Geometry check sheet. Reference: the model listing, model coordinates, mm. Face numbers are marked on the shaded views. A direction names the side the tool comes from. Round coordinates to 2 decimals unless told otherwise and drop trailing zeros. Write each loop counter-clockwise with the first axis right and the second up, starting at its lowest first coordinate (ties: lowest second). Pieces come first, ordered by that corner, then holes. Notation, with made-up numbers: M 57.5,-3 L 72.5,-3 A30 ccw 72.5,19 Z; hole C 53.25,-20 d5. An arc over 180 degrees is marked long. Put each result on its own line as item: value. Start each with the question number.
(1) Gauge pin test, flat ends, axial feed: pin 1 (11.5 mm diameter, centred on x = 48.26, z = -48.26, fed in from +Y); pin 2 (20.5 mm diameter, centred on x = 48.26, z = 48.26, fed in from +Y); pin 3 (19 mm diameter, centred on y = 23, z = -13, fed in from +X). Record the tip position at first contact, or that the pin passes through.
(2) Tool access check on the marked faces 1, 2 and 3. Record the directions out of +Z, -Z, +X, -X, +Y, -Y that give a thin tool (end or side, any length) a straight path to the whole face; none if there is none.
(3) Material ranges on probe 1 along Z at (x, y) = (48.26, -9.75); probe 2 along X at (y, z) = (45.5, 20), recorded low to high.
(4) Section check A-A on x = -48.26. Record the cut outline in (y, z).
(5) Section check C-C on z = -24. Record the cut outline in (x, y).
(6) Section check B-B on y = -9.5. Record the cut outline in (x, z), then the cut area to 3 significant figures.
(7) Mould release check, pull along Z, two halves, no side actions. Record for the marked faces 4, 5 and 6: pulls with the +Z half, pulls with the -Z half, needs draft (parallel to the pull), parting line crosses it, or undercut.
(8) Section check D-D on x = -21. Record the cut outline in (y, z).
from build123d import *

# Parameters (mm, degrees)
SKETCH1_W          = 127
SKETCH1_H          = 127
EXTRUDE1_DEPTH     = 19.05
EXTRUDE2_DEPTH     = 38.1
SKETCH3_R          = 12.7
CUT_EXTRUDE1_DEPTH = 38.1
SKETCH4_W          = 38.1
SKETCH4_H          = 63.5
CUT_EXTRUDE2_DEPTH = 38.1
CUT_EXTRUDE3_REACH = 21.05
SKETCH5_R          = 6.35
CUT_EXTRUDE4_REACH = 21.05
SKETCH6_R          = 6.35
CUT_EXTRUDE5_REACH = 21.05
SKETCH8_R          = 6.35


with BuildPart() as part:
    # Sketch1 → Extrude1 (new body)
    with BuildSketch(Plane(origin=(0, 0, 0), x_dir=(1, 0, 0), z_dir=(0, 1, 0))):
        Rectangle(SKETCH1_W, SKETCH1_H)
    extrude(amount=-EXTRUDE1_DEPTH)

    # Sketch2 → Extrude2 (add, symmetric)
    with BuildSketch(Plane(origin=(0, 0, 0), x_dir=(0, 0, -1), z_dir=(1, 0, 0))):
        Polygon((38.1, 0), (26.903236725, 63.5), (-26.903236725, 63.5), (-38.1, 0), align=None)
    extrude(amount=EXTRUDE2_DEPTH, both=True)

    # Sketch3 → Cut-Extrude1 (cut, symmetric)
    with BuildSketch(Plane(origin=(0, 0, 0), x_dir=(0, 0, -1), z_dir=(1, 0, 0))):
        with Locations((0, 31.75)):
            Circle(SKETCH3_R)
    extrude(amount=CUT_EXTRUDE1_DEPTH, both=True, mode=Mode.SUBTRACT)

    # Sketch4 → Cut-Extrude2 (cut, symmetric)
    with BuildSketch(Plane.XY):
        with Locations((0, 31.75)):
            Rectangle(SKETCH4_W, SKETCH4_H)
    extrude(amount=CUT_EXTRUDE2_DEPTH, both=True, mode=Mode.SUBTRACT)

    # Sketch5 → Cut-Extrude3 (cut, up to next)
    with BuildSketch(Plane(origin=(0, 0, 0), x_dir=(1, 0, 0), z_dir=(0, 1, 0)), mode=Mode.PRIVATE) as cut_extrude3_sk1:
        with Locations((-48.26, 48.26)):
            Circle(SKETCH5_R)
    cut_extrude3_tool1 = extrude(cut_extrude3_sk1.sketch, amount=-CUT_EXTRUDE3_REACH, mode=Mode.PRIVATE) & part.part
    add(cut_extrude3_tool1.solids().sort_by_distance((-48.26, 0, -48.26))[0], mode=Mode.SUBTRACT)

    # Sketch6 → Cut-Extrude4 (cut, up to next)
    with BuildSketch(Plane(origin=(0, 0, 0), x_dir=(1, 0, 0), z_dir=(0, 1, 0)), mode=Mode.PRIVATE) as cut_extrude4_sk1:
        with Locations((48.26, 48.26)):
            Circle(SKETCH6_R)
    cut_extrude4_tool1 = extrude(cut_extrude4_sk1.sketch, amount=-CUT_EXTRUDE4_REACH, mode=Mode.PRIVATE) & part.part
    add(cut_extrude4_tool1.solids().sort_by_distance((48.26, 0, -48.26))[0], mode=Mode.SUBTRACT)

    # Sketch8 → Cut-Extrude5 (cut, up to next)
    with BuildSketch(Plane(origin=(0, 0, 0), x_dir=(1, 0, 0), z_dir=(0, 1, 0)), mode=Mode.PRIVATE) as cut_extrude5_sk1:
        with Locations((-48.26, -48.26)):
            Circle(SKETCH8_R)
    cut_extrude5_tool1 = extrude(cut_extrude5_sk1.sketch, amount=-CUT_EXTRUDE5_REACH, mode=Mode.PRIVATE) & part.part
    add(cut_extrude5_tool1.solids().sort_by_distance((-48.26, 0, 48.26))[0], mode=Mode.SUBTRACT)
    # Sketch8 → Cut-Extrude5 (cut, up to next)
    with BuildSketch(Plane(origin=(0, 0, 0), x_dir=(1, 0, 0), z_dir=(0, 1, 0)), mode=Mode.PRIVATE) as cut_extrude5_sk2:
        with Locations((48.26, -48.26)):
            Circle(SKETCH8_R)
    cut_extrude5_tool2 = extrude(cut_extrude5_sk2.sketch, amount=-CUT_EXTRUDE5_REACH, mode=Mode.PRIVATE) & part.part
    add(cut_extrude5_tool2.solids().sort_by_distance((48.26, 0, 48.26))[0], mode=Mode.SUBTRACT)


solid = part.part
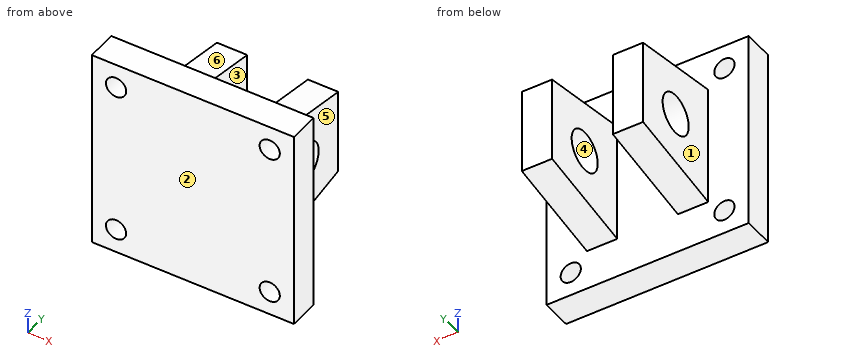
Answers follow:
1. pin 1: passes through
1. pin 2: stops at y = 0
1. pin 3: stops at x = 38.1
2. face 1: +Z, -Z, -X, +Y
2. face 2: +Z, -Z, +X, -X, -Y
2. face 3: +Z, -Z, +Y
3. probe 1: z = -63.5 to -54.61, -41.91 to 41.91, 54.61 to 63.5
3. probe 2: x = -38.1 to -19.05, 19.05 to 38.1
4. outline: M -19.05,-63.5 L 0,-63.5 L 0,-54.61 L -19.05,-54.61 Z; M -19.05,-41.91 L 0,-41.91 L 0,41.91 L -19.05,41.91 Z; M -19.05,54.61 L 0,54.61 L 0,63.5 L -19.05,63.5 Z
5. outline: M -63.5,-19.05 L 63.5,-19.05 L 63.5,0 L 38.1,0 L 38.1,63.5 L 19.05,63.5 L 19.05,0 L -19.05,0 L -19.05,63.5 L -38.1,63.5 L -38.1,0 L -63.5,0 Z
6. outline: M -63.5,-63.5 L 63.5,-63.5 L 63.5,63.5 L -63.5,63.5 Z; hole C -48.26,-48.26 d12.7; hole C -48.26,48.26 d12.7; hole C 48.26,-48.26 d12.7; hole C 48.26,48.26 d12.7
6. area: 15,600 mm^2
7. face 4: undercut
7. face 5: needs draft
7. face 6: pulls with the +Z half
8. outline: M -19.05,-63.5 L 0,-63.5 L 0,-38.1 L 63.5,-26.9 L 63.5,26.9 L 0,38.1 L 0,63.5 L -19.05,63.5 Z; hole C 31.75,0 d25.4
